Work out the finished part from the listing and answer in its coordinate system (mm). A direction names the side the tool comes from. Give positions to 0.01 mm unless a question says otherwise; leave off trailing zeros. Order: outer loops, then holes, each group sorted by start corner. A loop starts at its lowest first (then second) coordinate and runs counter-clockwise, first axis right, second up. Notation, with made-up numbers: (75, -25) - (127, -25) arc R18 cw to (127, 7) - close; hole circle Ø5 at (48, 56). An arc over 180 degrees is marked (long way). Put each result on its own line as item: value.
```python
from build123d import *

# Parameters (mm, degrees)
SKETCH_1_W               = 65
SKETCH_1_H               = 19
EXTRUDE_1_DEPTH          = 19
HOLE_WIZARD_M8_2_D       = 6.8
MM_2_D                   = 6
MM_2_DEPTH               = 20
MM_2_TIP                 = 1.802581857
SKETCH_6_W               = 79
SKETCH_6_H               = 19
EXTRUDE_2_DEPTH          = 60
MM_3_D                   = 6
HOLE_WIZARD_M6_1_D       = 5
CHAMFER_2_SIZE           = 30
CUT_EXTRUDE_1_DEPTH      = 118.249733475
CUT_EXTRUDE_2_DEPTH      = 124.118845024
CUT_EXTRUDE_2_DEPTH_BACK = 124.118845024


with BuildPart() as part:
    # 草图1 → 凸台-拉伸1 (new body)
    with BuildSketch(Plane(origin=(0, 0, 0), x_dir=(1, 0, 0), z_dir=(0, 1, 0))):
        Rectangle(SKETCH_1_W, SKETCH_1_H)
    extrude(amount=EXTRUDE_1_DEPTH)

    # M8 螺纹孔2 (through all)
    with Locations(Plane(origin=(0, 19, 0), x_dir=(1, 0, 0), z_dir=(0, 1, 0))):
        with Locations((-22.5, 0), (7.5, 0)):
            Hole(HOLE_WIZARD_M8_2_D / 2)

    # 大小mm 暗销孔2
    with Locations(Plane.XZ):
        with Locations((-7.5, 0), (22.5, 0)):
            Hole(MM_2_D / 2, depth=MM_2_DEPTH)
            with Locations((0, 0, -(MM_2_DEPTH + MM_2_TIP / 2))):  # 118° drill point
                Cone(0, MM_2_D / 2, MM_2_TIP, mode=Mode.SUBTRACT)

    # 草图6 → 凸台-拉伸2 (add)
    with BuildSketch(Plane(origin=(32.5, 0, 0), x_dir=(0, 0, -1), z_dir=(1, 0, 0))):
        with Locations((-30, 9.5)):
            Rectangle(SKETCH_6_W, SKETCH_6_H)
    extrude(amount=EXTRUDE_2_DEPTH)

    # 大小mm 暗销孔3 (through all)
    with Locations(Plane(origin=(0, 19, 0), x_dir=(1, 0, 0), z_dir=(0, 1, 0))):
        with Locations((86.5, -60), (66.5, -60)):
            Hole(MM_3_D / 2)

    # M6 螺纹孔1 (through all)
    with Locations(Plane(origin=(0, 19, 0), x_dir=(1, 0, 0), z_dir=(0, 1, 0))):
        with Locations((76.5, -60)):
            Hole(HOLE_WIZARD_M6_1_D / 2)

    # 倒角2
    chamfer_2_edges = [part.edges().sort_by_distance(p)[0] for p in [
        (32.5, 9.5, 9.5),
    ]]
    chamfer(chamfer_2_edges, length=CHAMFER_2_SIZE)

    # 草图11 → 切除-拉伸1 (cut, through all)
    with BuildSketch(Plane(origin=(0, 0, 0), x_dir=(-1, 0, 0), z_dir=(0, -1, 0))):
        Polygon((-51.5, -50.5), (-95.074786325, -50.5), (-95.074786325, 28.691704374), (-32.5, 28.691704374), (-32.5, -10.02428356), (-51.5, -29.02428356), align=None)
    extrude(amount=-CUT_EXTRUDE_1_DEPTH, mode=Mode.SUBTRACT)

    # 草图12 → 切除-拉伸2 (cut, two sides: drawn at the far end of the back side and taken through both)
    with BuildSketch(Plane.XY.offset(69.5).offset(-CUT_EXTRUDE_2_DEPTH_BACK)):
        Polygon((289.998105351, 184.165024638), (92.5, 13), (77.5, 0), (-119.998105351, -171.165024638), (222.331943924, -566.16123534), (632.328154627, -210.831186065), align=None)
    extrude(amount=CUT_EXTRUDE_2_DEPTH + CUT_EXTRUDE_2_DEPTH_BACK, mode=Mode.SUBTRACT)


solid = part.part
```
(1) Section C-C, the plane y = 15.5 is taken. Write down the section's boundary in (x, z).
Geometry check:
outline: (-32.5, -9.5) - (32.5, -9.5) - (32.5, 10.02) - (51.5, 29.02) - (51.5, 50.5) - (92.5, 50.5) - (92.5, 69.5) - (32.5, 69.5) - (32.5, 39.5) - (2.5, 9.5) - (-32.5, 9.5) - close; hole circle Ø6.8 at (-22.5, 0); hole circle Ø6 at (-7.5, 0); hole circle Ø6.8 at (7.5, 0); hole circle Ø6 at (22.5, 0); hole circle Ø6 at (66.5, 60); hole circle Ø5 at (76.5, 60); hole circle Ø6 at (86.5, 60)
(2) Section B-B, the plane z = 0 is taken. Write down the section's boundary in (x, y), then the cut area to 3 significant figures.
Geometry check:
outline: (-32.5, 0) - (-25.9, 0) - (-25.9, 19) - (-32.5, 19) - close; (-19.1, 0) - (-10.5, 0) - (-10.5, 19) - (-19.1, 19) - close; (-4.5, 0) - (4.1, 0) - (4.1, 19) - (-4.5, 19) - close; (10.9, 0) - (19.5, 0) - (19.5, 19) - (10.9, 19) - close; (25.5, 0) - (32.5, 0) - (32.5, 19) - (25.5, 19) - close
area: 749 mm²
(3) Given pin 1 (12 mm diameter, centred on x = 45.5, z = 10, fed in from +Y); pin 2 (5.5 mm diameter, centred on x = 80, y = 12, fed in from -Z); pin 3 (5 mm diameter, centred on y = 6.5, z = 2, fed in from +X); pin 4 (5.5 mm diameter, centred on x = -21.5, y = 13, fed in from +Z), each flat-ended and moving along its own axis, determine where each tip first touches the part or whether it passes through.
Geometry check:
pin 1: passes through
pin 2: stops at z = 50.5
pin 3: stops at x = 32.5
pin 4: stops at z = 9.5
(4) A tool of negligible diameter and unlimited length cuts with its end or side. For faces 4 (the face through (32.5, 10, 55)), 5 (the face through (-32.5, 9, 0)), 6 (the face through (72, 9, 50.5)), from which of +Z, -Z, +X, -X, +Y, -Y can it reach the whole face along a straight path? Write none if from no direction.
Geometry check:
face 4: +Z, -X, +Y, -Y
face 5: +Z, -Z, -X, +Y, -Y
face 6: -Z, +X, +Y, -Y
(5) Determine the mould class of faces 1 (the face through (68.71, 9.37, 57.97)), 2 (the face through (83.44, 5.15, 61.98)), 3 (the face through (0, 9, -9.5)) for opening direction Z: pulls with the +Z half, pulls with the -Z half, needs draft (parallel to the pull), parting line crosses it, or undercut.
Geometry check:
face 1: undercut
face 2: needs draft
face 3: pulls with the -Z half
(6) Straight lines are drawn through the part: line 1 (Z direction, x = 76.5, y = 8.75); line 2 (X direction, y = 13, z = -1); line 3 (X direction, y = 2, z = -4). For each, find the intervals that lie inside material, in ascending order.
Geometry check:
line 1: z = 50.5 to 57.5, 62.5 to 69.5
line 2: x = -32.5 to -25.75, -19.25 to -10.33, -4.67 to 4.25, 10.75 to 19.67, 25.33 to 32.5
line 3: x = -32.5 to 32.5
(7) Section D-D, the plane x = -22.5 is taken. Write down the section's boundary in (y, z).
Geometry check:
outline: (0, -9.5) - (19, -9.5) - (19, -3.4) - (0, -3.4) - close; (0, 3.4) - (19, 3.4) - (19, 9.5) - (0, 9.5) - close
(8) Section A-A, the plane x = 7.5 is taken. Write down the section's boundary in (y, z), then the cut area to 3 significant figures.
Geometry check:
outline: (0, -9.5) - (19, -9.5) - (19, -3.4) - (0, -3.4) - close; (0, 3.4) - (19, 3.4) - (19, 14.5) - (0, 14.5) - close
area: 327 mm²
